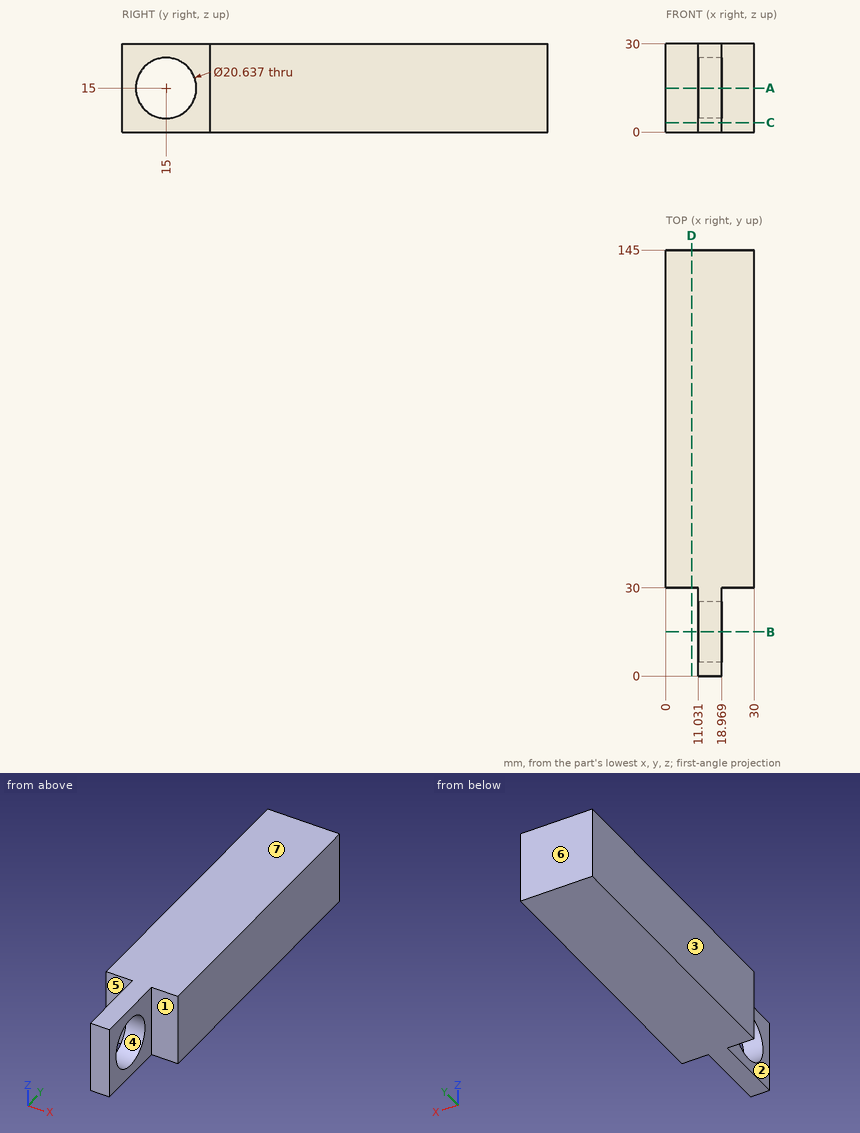
Answer from the drawing. Dimensions are ordinates in mm from the lowest x, y and z of the part. A direction names the side the tool comes from. Coordinates: 2 decimals unless noted, no trailing zeros. Order: outer loops, then holes, each group sorted by start corner. A loop starts at its lowest first (then second) coordinate and runs counter-clockwise, first axis right, second up. Notation, with made-up numbers: (-15.5, -18) - (-1.5, -18) arc R32 ccw to (-1.5, 20) - close; hole circle Ø9 at (-28.5, 6.5). An arc over 180 degrees is marked (long way). Put each result on its own line as item: value. Start each with the question number.
1) For the marked faces 1, 2 and 3, determine the directions among +Z, -Z, +X, -X, +Y, -Y from which every point of the face is accessible in a straight line to the end or side of a thin tool.
2) Find section A-A (z = 15). Give the vertices of the cut face in (x, y).
3) A flat-ended cylindrical pin translates along its axis: pin 1 (9 mm diameter, centred on x = 25, z = 13.5, fed in from -Y). Find the tip coordinate at first contact, or state that the pin passes through.
4) Find the intervals of material crossed by line 1 (Z direction, x = 15.25, y = 15); line 2 (Y direction, x = 20.5, z = 9); line 3 (Y direction, x = 14.75, z = 10.25), in increasing order. Write a range as from..to.
5) Find section C-C (z = 3.25). Give the vertices of the cut face in (x, y).
6) Find section B-B (y = 15). Give the vertices of the cut face in (x, z).
7) Find section D-D (x = 8.75). Give the vertices of the cut face in (y, z), plus the area to 3 significant figures.
8) For a pull along Y with two mould halves and no side action, classify the marked faces 4, 5, 6 and 7 as released by +Y, released by -Y, zero draft, split by the parting line, or undercut.
Results list:
1. face 1: +Z, -Z, +X, -Y
1. face 2: +Z, -Z, -X, -Y
1. face 3: +Z, -Z, -X, +Y, -Y
2. outline: (0, 30) - (11.03, 30) - (11.03, 25.32) - (18.97, 25.32) - (18.97, 30) - (30, 30) - (30, 145) - (0, 145) - close; (11.03, 0) - (18.97, 0) - (18.97, 4.68) - (11.03, 4.68) - close
3. pin 1: stops at y = 30
4. line 1: z = 0..4.68, 25.32..30
4. line 2: y = 30..145
4. line 3: y = 0..5.84, 24.16..145
5. outline: (0, 30) - (11.03, 30) - (11.03, 0) - (18.97, 0) - (18.97, 30) - (30, 30) - (30, 145) - (0, 145) - close
6. outline: (11.03, 0) - (18.97, 0) - (18.97, 4.68) - (11.03, 4.68) - close; (11.03, 25.32) - (18.97, 25.32) - (18.97, 30) - (11.03, 30) - close
7. outline: (30, 0) - (145, 0) - (145, 30) - (30, 30) - close
7. area: 3,450 mm^2
8. face 4: undercut
8. face 5: released by -Y
8. face 6: released by +Y
8. face 7: zero draft
